Part print with two shaded views. Sizes in mm from the minimum x, y, z corner. Round coordinates to 2 decimals unless told otherwise and drop trailing zeros. Write each loop counter-clockwise with the first axis right and the second up, starting at its lowest first coordinate (ties: lowest second). Pieces come first, ordered by that corner, then holes. Notation, with made-up numbers: (6, 54.5) -> (25, 54.5) arc R26 cw to (25, 81.5) -> close; hole circle Ø8 at (74.5, 59). An arc over 180 degrees is marked (long way). Return JSON: item names as keys, results as strings. Group by question number.
(1) Saw through at A-A (z = 31). List the corners of the cut face in (x, y).
(2) Drill centre lines: L1, parallel to X at y = 2.45, z = 47; L2, parallel to X at y = 0.2, z = 37; L3, parallel to Z at x = 82, y = 1.55. Where is each one in solid material? Low to high. Write a range as from..to.
(3) Saw through at B-B (x = 80.5). List the corners of the cut face in (y, z).
(4) Drop flat-ended pins along their axis: pin 1 Ø1.5 at (x, y) = (84.5, 2) entering from +Z; pin 2 Ø0.9 at (y, z) = (2, 13) entering from +X. Give the stop position or say it passes through.
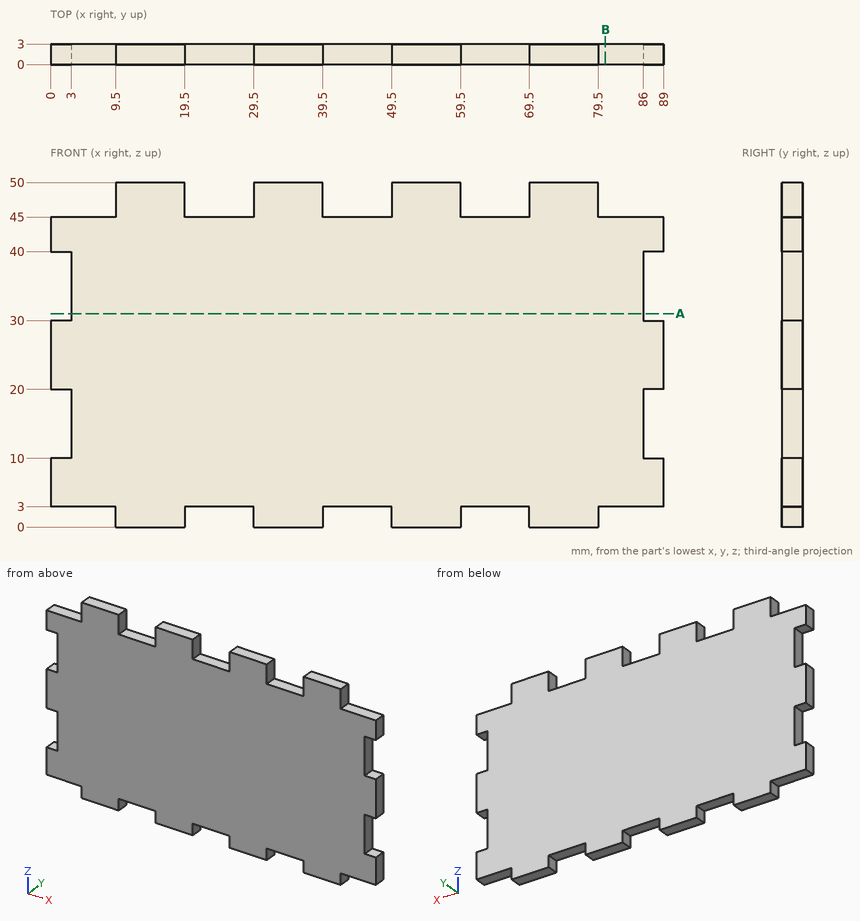
Computed values:
{
 "1": {"outline": "(3, 0) -> (86, 0) -> (86, 3) -> (3, 3) -> close"},
 "2": {"L1": "9.5..19.5, 29.5..39.5, 49.5..59.5, 69.5..79.5", "L2": "3..86", "L3": "3..45"},
 "3": {"outline": "(0, 3) -> (3, 3) -> (3, 45) -> (0, 45) -> close"},
 "4": {"pin 1": "z = 45", "pin 2": "x = 86"}
}
